Design review of the part built by this model. Coordinates are the model's own, in mm. A direction names the side the tool comes from. Coordinates: 2 decimals unless noted, no trailing zeros. Order: outer loops, then holes, each group sorted by start corner. A loop starts at its lowest first (then second) coordinate and runs counter-clockwise, first axis right, second up. Notation, with made-up numbers: M 43.5,89.5 L 74.5,89.5 A31 cw 74.5,119.5 Z; hole C -20,-1 d10. An arc over 180 degrees is marked long. Answer as a JSON object with one key per item and string values.
from build123d import *

# Parameters (mm, degrees)
ESQUISSE1_W                  = 9
ESQUISSE1_H                  = 45
ESQUISSE1_W_2                = 5.6
ESQUISSE1_H_2                = 2.6
BOSS_EXTRU_1_DEPTH           = 1.25
ENL_V_MAT_EXTRU_1_DEPTH      = 44.859616193
ENL_V_MAT_EXTRU_1_DEPTH_BACK = 44.859616193
ESQUISSE2_W                  = 2.5
ESQUISSE2_H                  = 4.5
ESQUISSE3_W                  = 5.6
ESQUISSE3_H                  = 1
BOSS_EXTRU_2_DEPTH           = 1.5


with BuildPart() as part:
    # Esquisse1 → Boss.-Extru.1 (new body)
    with BuildSketch(Plane(origin=(0, 0, 0), x_dir=(1, 0, 0), z_dir=(0, 1, 0))):
        with Locations((3.408982136, 20.622516556)):
            Rectangle(ESQUISSE1_W, ESQUISSE1_H)
        with Locations((3.408982136, 35.822516556)):
            Rectangle(ESQUISSE1_W_2, ESQUISSE1_H_2, mode=Mode.SUBTRACT)
        with Locations((3.408982136, 5.422516556)):
            Rectangle(ESQUISSE1_W_2, ESQUISSE1_H_2, mode=Mode.SUBTRACT)
    extrude(amount=BOSS_EXTRU_1_DEPTH)

    # Esquisse2 → Enlèv. mat.-Extru.1 (cut, two sides: drawn at the far end of the back side and taken through both)
    with BuildSketch(Plane.XZ.offset(-ENL_V_MAT_EXTRU_1_DEPTH_BACK)):
        with Locations((3.408982136, -20.622516556)):
            Rectangle(ESQUISSE2_W, ESQUISSE2_H)
    extrude(amount=ENL_V_MAT_EXTRU_1_DEPTH + ENL_V_MAT_EXTRU_1_DEPTH_BACK, mode=Mode.SUBTRACT)

    # Esquisse3 → Boss.-Extru.2 (add)
    with BuildSketch(Plane(origin=(0, 1.25, 0), x_dir=(1, 0, 0), z_dir=(0, 1, 0))):
        with Locations((3.408982136, 7.222516556)):
            Rectangle(ESQUISSE3_W, ESQUISSE3_H)
        with Locations((3.408982136, 34.022516556)):
            Rectangle(ESQUISSE3_W, ESQUISSE3_H)
    extrude(amount=BOSS_EXTRU_2_DEPTH)


solid = part.part
1) Add section C-C (z = -20). State the section outline as (x, y) points.
Taken from the geometry:
{"outline": "M -1.09,0 L 2.16,0 L 2.16,1.25 L -1.09,1.25 Z; M 4.66,0 L 7.91,0 L 7.91,1.25 L 4.66,1.25 Z"}
2) Add section D-D (x = 3). State the section outline as (y, z) points, and give its area (3 significant figures).
Taken from the geometry:
{"outline": "M 0,-43.12 L 1.25,-43.12 L 1.25,-37.12 L 0,-37.12 Z; M 0,-34.52 L 2.75,-34.52 L 2.75,-33.52 L 1.25,-33.52 L 1.25,-22.87 L 0,-22.87 Z; M 0,-18.37 L 1.25,-18.37 L 1.25,-7.72 L 2.75,-7.72 L 2.75,-6.72 L 0,-6.72 Z; M 0,-4.12 L 1.25,-4.12 L 1.25,1.88 L 0,1.88 Z", "area": "47.1 mm2"}
3) Tool access review of faces 1 (the flat face through (0.609, 2, -34)), 2 (the flat face through (6.209, 2, -34)), 3 (the flat face through (-1.091, 1, -20)), 4 (the flat face through (3, 1, -37.123)), 5 (the flat face through (3, 2, -7.723)): name each direction out of +Z, -Z, +X, -X, +Y, -Y from which nothing blocks a thin tool from reaching the whole face with its end or side.
Taken from the geometry:
{"face 1": "+Z, -Z, -X, +Y", "face 2": "+Z, -Z, +X, +Y", "face 3": "+Z, -Z, -X, +Y, -Y", "face 4": "+Y, -Y", "face 5": "+X, -X, +Y"}
4) Add section A-A (x = 5.5). State the section outline as (y, z) points, and give its area (4 significant figures).
Taken from the geometry:
{"outline": "M 0,-43.12 L 1.25,-43.12 L 1.25,-37.12 L 0,-37.12 Z; M 0,-34.52 L 2.75,-34.52 L 2.75,-33.52 L 1.25,-33.52 L 1.25,-7.72 L 2.75,-7.72 L 2.75,-6.72 L 0,-6.72 Z; M 0,-4.12 L 1.25,-4.12 L 1.25,1.88 L 0,1.88 Z", "area": "52.75 mm2"}
5) Mouldability with a two-part tool opening along X and no side actions: class faces 6 (the flat face through (6.209, 2, -7)), 7 (the flat face through (3, 1, -34.523)), 8 (the flat face through (3, 2, -33.523)) as released by +X, released by -X, zero draft, split by the parting line, or undercut.
Taken from the geometry:
{"face 6": "released by +X", "face 7": "undercut", "face 8": "zero draft"}
6) Insertion check: pin 1 Ø0.5 at (y, z) = (2.5, -7) entering from -X; pin 2 Ø0.5 at (y, z) = (2, -7.5) entering from +X; pin 3 Ø1.4 at (x, y) = (4, 2) entering from -Z; pin 4 Ø1 at (x, z) = (4, -7) entering from -Y. Each pin has a flat end and moves straight along its axis. Give the tip position at first contact, or say it passes through.
Taken from the geometry:
{"pin 1": "stops at x = 0.61", "pin 2": "stops at x = 6.21", "pin 3": "stops at z = -34.52", "pin 4": "stops at y = 0"}
7) Add section B-B (y = 1.7). State the section outline as (x, z) points.
Taken from the geometry:
{"outline": "M 0.61,-34.52 L 6.21,-34.52 L 6.21,-33.52 L 0.61,-33.52 Z; M 0.61,-7.72 L 6.21,-7.72 L 6.21,-6.72 L 0.61,-6.72 Z"}
8) To check wall thickness, follow L1, parallel to Z at x = 5.25, y = 0.4; L2, parallel to Z at x = 0.75, y = 2.65; L3, parallel to Y at x = -0.25, z = -10.5. State the ranges of each line that lie inside material, in increasing order.
Taken from the geometry:
{"L1": "z = -43.12 to -37.12, -34.52 to -6.72, -4.12 to 1.88", "L2": "z = -34.52 to -33.52, -7.72 to -6.72", "L3": "y = 0 to 1.25"}
